from build123d import *

# Parameters (mm, degrees)
F0_W     = 32
F0_H     = 32
F0_R     = 2
F1_DEPTH = 5
F2_W     = 70
F2_H     = 30
F2_R     = 2
F2_R_2   = 5
F3_DEPTH = 3


with BuildPart() as f1:
    # F0 (on Top) → F1 (new body)
    with BuildSketch(Plane.XY):
        Rectangle(F0_W, F0_H)
        with Locations((-10, -10)):
            Circle(F0_R, mode=Mode.SUBTRACT)
        with Locations((10, -10)):
            Circle(F0_R, mode=Mode.SUBTRACT)
        with Locations((-10, 10)):
            Circle(F0_R, mode=Mode.SUBTRACT)
        with Locations((10, 10)):
            Circle(F0_R, mode=Mode.SUBTRACT)
    extrude(amount=F1_DEPTH)

    # F2 (on Front) → F3 (join, symmetric)
    with BuildSketch(Plane.XZ):
        with Locations((5, 15)):
            Rectangle(F2_W, F2_H)
        with Locations((-15, 10.25)):
            Circle(F2_R, mode=Mode.SUBTRACT)
        with Locations((-23, 18.25)):
            Circle(F2_R, mode=Mode.SUBTRACT)
        with Locations((-15, 18.25)):
            Circle(F2_R_2, mode=Mode.SUBTRACT)
        with Locations((-7, 18.25)):
            Circle(F2_R, mode=Mode.SUBTRACT)
        with Locations((-15, 26.25)):
            Circle(F2_R, mode=Mode.SUBTRACT)
        with Locations((34, 20)):
            Circle(F2_R, mode=Mode.SUBTRACT)
    extrude(amount=F3_DEPTH, both=True)


solid = f1.part
Geometry: final body of the model. Coordinates: model frame, mm. A direction names the side the tool comes from. Round coordinates to 2 decimals unless told otherwise and drop trailing zeros. Loops run counter-clockwise (first coordinate to the right, second up) from the corner with the lowest first, then second, coordinate; pieces in that order, holes last. Notation, with made-up numbers: (51.25, 56.25) - (55.25, 56.25) arc R16 ccw to (55.25, 83.25) - close; hole circle Ø9 at (16.25, 59.5). An arc over 180 degrees is marked (long way). Write each question's results on one line, items separated by ' | '. Start each with the question number.
1) Line query: probe 1 along Y at (x, z) = (10, 3.3); probe 2 along Z at (x, y) = (-15, -1.8); probe 3 along X at (y, z) = (-1.5, 16.5). Output: solid intervals per line, ascending. Write a range as [from, to].
2) First-contact query: P1, Ø9, axis at x = -9.5, z = 20, coming from the -Y side; P2, Ø14.5, axis at x = -4, y = -10.5, coming from the +Z side; P3, Ø5, axis at x = -7.5, z = 10, coming from the +Y side. Flat tips, straight axial feed; report the tip coordinate or a pass-through.
3) Cut plane D-D on z = 19.25. Return loops of the section in (x, y), then the cut area to 3 significant figures.
4) Cut plane B-B on y = 2. Return loops of the section in (x, z), then the cut area to 3 significant figures.
5) Access query for faces 1 (the face through (-16, 9, 2)), 2 (the face through (40, 0, 15)), 3 (the face through (0, -9, 5)). Directions: +Z, -Z, +X, -X, +Y, -Y. A direction counts if a zero-diameter tool reaches every point of the face in a straight line with its end or side. Return the directions, or none.
6) Mould query, pull axis X, two halves, no side actions, for faces 4 (the face through (16, -10, 2)), 5 (the face through (-16.08, 0.04, 13.37)), 6 (the face through (-16, -10, 2)). Classes: released by +X, released by -X, zero draft, split by the parting line, or undercut.
7) Cut plane C-C on x = 10. Return loops of the section in (y, z), then the cut area to 3 significant figures.
8) Cut plane A-A on x = -23. Return loops of the section in (y, z), then the cut area to 3 significant figures.
Verdict:
1) probe 1: y = [-16, -12], [-8, 8], [12, 16] | probe 2: z = [0, 8.25], [12.25, 13.25], [23.25, 24.25], [28.25, 30] | probe 3: x = [-30, -23.97], [-22.03, -19.68], [-10.32, -7.97], [-6.03, 40]
2) P1: stops at y = -3 | P2: stops at z = 5 | P3: stops at y = 3
3) outline: (-30, -3) - (-24.73, -3) - (-24.73, 3) - (-30, 3) - close; (-21.27, -3) - (-19.9, -3) - (-19.9, 3) - (-21.27, 3) - close; (-10.1, -3) - (-8.73, -3) - (-8.73, 3) - (-10.1, 3) - close; (-5.27, -3) - (32.15, -3) - (32.15, 3) - (-5.27, 3) - close; (35.85, -3) - (40, -3) - (40, 3) - (35.85, 3) - close | area: 297 mm2
4) outline: (-30, 0) - (40, 0) - (40, 30) - (-30, 30) - close; hole circle Ø4 at (-23, 18.25); hole circle Ø10 at (-15, 18.25); hole circle Ø4 at (-15, 10.25); hole circle Ø4 at (-15, 26.25); hole circle Ø4 at (-7, 18.25); hole circle Ø4 at (34, 20) | area: 1,960 mm2
5) face 1: +Z, -Z, -X, +Y | face 2: +Z, -Z, +X, +Y, -Y | face 3: +Z, +X, -X, -Y
6) face 4: released by +X | face 5: undercut | face 6: released by -X
7) outline: (-16, 0) - (-12, 0) - (-12, 5) - (-16, 5) - close; (-8, 0) - (8, 0) - (8, 5) - (3, 5) - (3, 30) - (-3, 30) - (-3, 5) - (-8, 5) - close; (12, 0) - (16, 0) - (16, 5) - (12, 5) - close | area: 270 mm2
8) outline: (-3, 0) - (3, 0) - (3, 16.25) - (-3, 16.25) - close; (-3, 20.25) - (3, 20.25) - (3, 30) - (-3, 30) - close | area: 156 mm2
